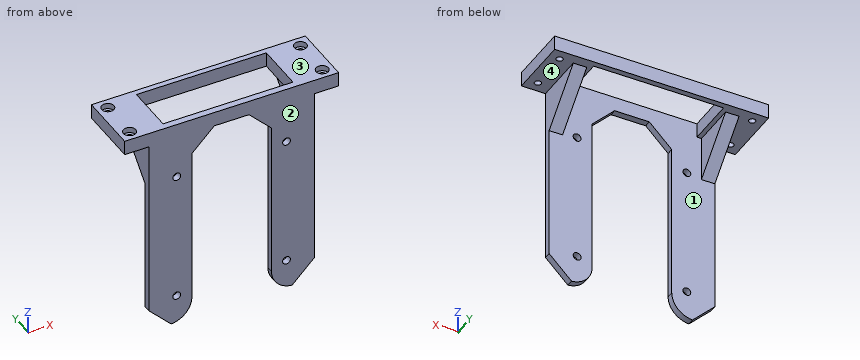
```python
from build123d import *

# Parameters (mm, degrees)
SKETCH1_W                        = 95.5
SKETCH1_H                        = 27.5
BOSS_EXTRUDE1_DEPTH              = 6.5
SKETCH2_W                        = 74
SKETCH2_H                        = 3
BOSS_EXTRUDE2_DEPTH              = 90
SKETCH3_W                        = 58
SKETCH3_H                        = 22
CUT_EXTRUDE1_DEPTH               = 90
CBORE_FOR_M2_5_SHCS1_D           = 2.9
CBORE_FOR_M2_5_SHCS1_DEPTH       = 10.1
CBORE_FOR_M2_5_SHCS1_CBORE_D     = 5.5
CBORE_FOR_M2_5_SHCS1_CBORE_DEPTH = 2.5
CBORE_FOR_M2_5_SHCS1_TIP         = 0.871247898
SKETCH7_W                        = 6
SKETCH7_H                        = 20
BOSS_EXTRUDE3_DEPTH              = 20
CHAMFER1_SIZE                    = 20
F_1_0_3_5_DIAMETER_HOLE1_D       = 3.5
F_1_0_3_5_DIAMETER_HOLE1_DEPTH   = 10.1
F_1_0_3_5_DIAMETER_HOLE1_TIP     = 1.051506083
SKETCH12_W                       = 35.5
SKETCH12_H                       = 90
CUT_EXTRUDE2_DEPTH               = 20
CHAMFER2_SIZE                    = 10
FILLET1_R                        = 10


# Some blends are built 0.0001 mm under size
with BuildPart() as part:
    # Sketch1 → Boss-Extrude1 (new body)
    with BuildSketch(Plane.XY):
        Rectangle(SKETCH1_W, SKETCH1_H)
    extrude(amount=BOSS_EXTRUDE1_DEPTH)

    # Sketch2 → Boss-Extrude2 (add)
    with BuildSketch(Plane(origin=(0, 0, 0), x_dir=(-1, 0, 0), z_dir=(0, 0, -1))):
        with Locations((0, -12.25)):
            Rectangle(SKETCH2_W, SKETCH2_H)
    extrude(amount=BOSS_EXTRUDE2_DEPTH)

    # Sketch3 → Cut-Extrude1 (cut)
    with BuildSketch(Plane(origin=(0, 0, 0), x_dir=(-1, 0, 0), z_dir=(0, 0, -1))):
        with Locations((0, 0.25)):
            Rectangle(SKETCH3_W, SKETCH3_H)
    extrude(amount=-CUT_EXTRUDE1_DEPTH, mode=Mode.SUBTRACT)

    # CBORE for M2.5 SHCS1
    with Locations(Plane.XY.offset(6.5)):
        with Locations((-43, 9), (-43, -9), (43, 9), (43, -9)):
            CounterBoreHole(CBORE_FOR_M2_5_SHCS1_D / 2, CBORE_FOR_M2_5_SHCS1_CBORE_D / 2, CBORE_FOR_M2_5_SHCS1_CBORE_DEPTH, depth=CBORE_FOR_M2_5_SHCS1_DEPTH)
            with Locations((0, 0, -(CBORE_FOR_M2_5_SHCS1_DEPTH + CBORE_FOR_M2_5_SHCS1_TIP / 2))):  # 118° drill point
                Cone(0, CBORE_FOR_M2_5_SHCS1_D / 2, CBORE_FOR_M2_5_SHCS1_TIP, mode=Mode.SUBTRACT)

    # Sketch7 → Boss-Extrude3 (add)
    with BuildSketch(Plane(origin=(0, 0, 0), x_dir=(-1, 0, 0), z_dir=(0, 0, -1))):
        with Locations((-34, -0.75)):
            Rectangle(SKETCH7_W, SKETCH7_H)
        with Locations((34, -0.75)):
            Rectangle(SKETCH7_W, SKETCH7_H)
    extrude(amount=BOSS_EXTRUDE3_DEPTH)

    # Chamfer1
    chamfer1_edges = [part.edges().sort_by_distance(p)[0] for p in [
        (34, 9.25, -20),
        (-34, 9.25, -20),
    ]]
    chamfer(chamfer1_edges, length=CHAMFER1_SIZE - 0.0001)  # a hair under: the kernel refuses the full size

    # Ø1.0 (3.5) Diameter Hole1
    with Locations(Plane(origin=(0, -10.75, 0), x_dir=(1, 0, 0), z_dir=(0, 1, 0))):
        with Locations((-24.5, 77), (24.5, 77), (-24.5, 19), (24.5, 19)):
            Hole(F_1_0_3_5_DIAMETER_HOLE1_D / 2, depth=F_1_0_3_5_DIAMETER_HOLE1_DEPTH)
            with Locations((0, 0, -(F_1_0_3_5_DIAMETER_HOLE1_DEPTH + F_1_0_3_5_DIAMETER_HOLE1_TIP / 2))):  # 118° drill point
                Cone(0, F_1_0_3_5_DIAMETER_HOLE1_D / 2, F_1_0_3_5_DIAMETER_HOLE1_TIP, mode=Mode.SUBTRACT)

    # Sketch12 → Cut-Extrude2 (cut)
    with BuildSketch(Plane(origin=(0, -10.75, 0), x_dir=(1, 0, 0), z_dir=(0, 1, 0))):
        with Locations((0, 45)):
            Rectangle(SKETCH12_W, SKETCH12_H)
    extrude(amount=-CUT_EXTRUDE2_DEPTH, mode=Mode.SUBTRACT)

    # Chamfer2
    chamfer2_edges = [part.edges().sort_by_distance(p)[0] for p in [
        (17.75, -12.25, 0),
        (-17.75, -12.25, 0),
        (37, -12.25, -90),
        (-37, -12.25, -90),
    ]]
    chamfer(chamfer2_edges, length=CHAMFER2_SIZE)

    # Fillet1
    # the kernel refuses this fillet: 10 mm, written as the material it takes off along each edge
    with BuildSketch(Plane(origin=(-17.75, 14.179588344, -90), x_dir=(0, 0, 1), z_dir=(0, -1, 0))) as fillet1_piece_1:
        with BuildLine():
            CenterArc((9.971835338, 10), FILLET1_R, 184.301222305, 85.698777695)
            Line((0, 9.25), (-0.199436707, 9.235))
            ThreePointArc((-0.199436707, 9.235), (-0.2, 4.625), (-0.2, 0))
            Line((-0.2, 0), (0, -0.2))
            Line((0, -0.2), (9.971835338, -0.2))
            Line((9.971835338, -0.2), (9.971835338, 0))
        make_face()
    extrude(amount=52.859176688, mode=Mode.SUBTRACT)
    with BuildSketch(Plane(origin=(17.75, 14.179588344, -90), x_dir=(1, 0, 0), z_dir=(0, -1, 0))) as fillet1_piece_2:
        with BuildLine():
            CenterArc((10, 9.971835338), FILLET1_R, 180, 85.698777695)
            Line((0, 9.971835338), (-0.2, 9.971835338))
            Line((-0.2, 9.971835338), (-0.2, 0))
            Line((-0.2, 0), (0, -0.2))
            ThreePointArc((0, -0.2), (4.625, -0.2), (9.235, -0.199436707))
            Line((9.235, -0.199436707), (9.25, 0))
        make_face()
    extrude(amount=52.859176688, mode=Mode.SUBTRACT)


solid = part.part
```
Geometry: final body of the model. Coordinates: model frame, mm. Face numbers are marked on the shaded views. A direction names the side the tool comes from. Round coordinates to 2 decimals unless told otherwise and drop trailing zeros. Order: outer loops, then holes, each group sorted by start corner. A loop starts at its lowest first (then second) coordinate and runs counter-clockwise, first axis right, second up. Notation, with made-up numbers: (0.25, 14.25) -> (36.25, 14.25) arc R17 ccw to (36.25, 24.25) -> close; hole circle Ø2 at (-4.75, 65). An arc over 180 degrees is marked (long way). Use CSV: the item, a comma, the result in double quotes. Start each with the question number.
1) Section A-A (z = -40). Return the cut outline in (x, y).
2) Section B-B (x = -43). Return the cut outline in (y, z), and give its area (3 significant figures).
3) Material intervals for line 1 along Y through (x, z) = (43, 5.3); line 2 along Y through (x, z) = (43, 2); line 3 along X through (y, z) = (1.25, 2), sorted ascending. Write a range as from..to.
4) First-contact query: pin 1 Ø1.5 at (y, z) = (-12, -42) entering from -X; pin 2 Ø4.5 at (x, z) = (-24.5, -77) entering from +Y; pin 3 Ø3.5 at (y, z) = (-13, -57) entering from +X; pin 4 Ø2 at (x, y) = (-24.5, -9.5) entering from +Z. Flat tips, straight axial feed; report the tip coordinate or a pass-through.
5) Section C-C (y = 2.25). Return the cut outline in (x, z).
6) Draft query along X for the marked faces 1 and 2. Return one class per face: +X half, -X half, draft (parallel to the pull), parting line (faces both ways), or undercut.
7) Section D-D (z = -77). Return the cut outline in (x, y), and give its area (3 significant figures).
8) Set-up query: the marked faces 3 and 4. Return all of +Z, -Z, +X, -X, +Y, -Y with unobstructed straight access to the full face (end or side cutting, diameter ignored); none if empty.
Returned:
1,outline,"(-37, -13.75) -> (-17.75, -13.75) -> (-17.75, -10.75) -> (-37, -10.75) -> close; (17.75, -13.75) -> (37, -13.75) -> (37, -10.75) -> (17.75, -10.75) -> close"
2,outline,"(-13.75, 0) -> (-10.45, 0) -> (-10.45, 4) -> (-11.75, 4) -> (-11.75, 6.5) -> (-13.75, 6.5) -> close; (-7.55, 0) -> (7.55, 0) -> (7.55, 4) -> (6.25, 4) -> (6.25, 6.5) -> (-6.25, 6.5) -> (-6.25, 4) -> (-7.55, 4) -> close; (10.45, 0) -> (13.75, 0) -> (13.75, 6.5) -> (11.75, 6.5) -> (11.75, 4) -> (10.45, 4) -> close"
2,area,"128 mm²"
3,line 1,"y = -13.75..-11.75, -6.25..6.25, 11.75..13.75"
3,line 2,"y = -13.75..-10.45, -7.55..7.55, 10.45..13.75"
3,line 3,"x = -47.75..-29, 29..47.75"
4,pin 1,"stops at x = -37"
4,pin 2,"stops at y = -10.75"
4,pin 3,"stops at x = 37"
4,pin 4,"passes through"
5,outline,"(-47.75, 0) -> (-37, 0) -> (-37, -7) -> (-31, -7) -> (-31, 0) -> (-29, 0) -> (-29, 6.5) -> (-47.75, 6.5) -> close; (29, 0) -> (31, 0) -> (31, -7) -> (37, -7) -> (37, 0) -> (47.75, 0) -> (47.75, 6.5) -> (29, 6.5) -> close"
6,face 1,"undercut"
6,face 2,"draft"
7,outline,"(-37, -13.75) -> (-26.25, -13.75) -> (-26.25, -10.75) -> (-37, -10.75) -> close; (-22.75, -13.75) -> (-17.75, -13.75) -> (-17.75, -10.75) -> (-22.75, -10.75) -> close; (17.75, -13.75) -> (22.75, -13.75) -> (22.75, -10.75) -> (17.75, -10.75) -> close; (26.25, -13.75) -> (37, -13.75) -> (37, -10.75) -> (26.25, -10.75) -> close"
7,area,"94.5 mm²"
8,face 3,"+Z, +X, -X, +Y, -Y"
8,face 4,"-Z, +Y"
